Input: part model. Units: mm. Frame: model coordinates. Face numbers are marked on the shaded views. Coordinates: 2 decimals unless noted, no trailing zeros. Order: outer loops, then holes, each group sorted by start corner. A loop starts at its lowest first (then second) coordinate and runs counter-clockwise, first axis right, second up. Notation, with made-up numbers: (69, -31) - (93, -31) arc R21 ccw to (93, -22) - close; hole circle Ø5 at (57.5, 35.5). An arc over 180 degrees is marked (long way). Use a Markdown table: item, result. Add a question column.
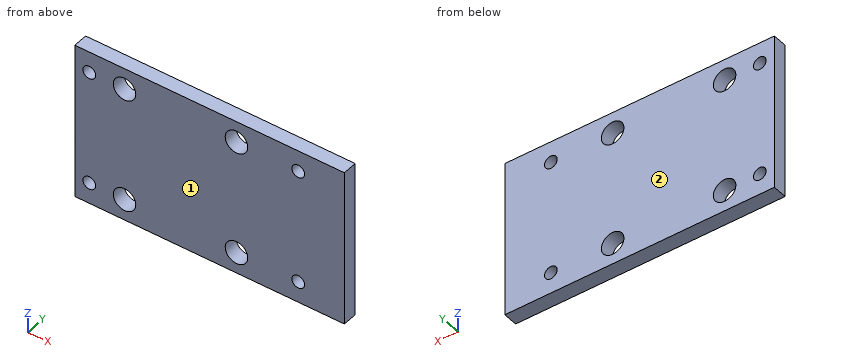
from build123d import *

# Parameters (mm, degrees)
SKETCH1_W           = 74.2
SKETCH1_H           = 46
BOSS_EXTRUDE1_DEPTH = 43
SKETCH2_R           = 11.5
SKETCH2_R_2         = 1.75
SKETCH2_R_3         = 2.5
CUT_EXTRUDE1_DEPTH  = 20
SKETCH3_R           = 3.1
SKETCH3_R_2         = 1.75
CUT_EXTRUDE2_DEPTH  = 15
CUT_EXTRUDE3_DEPTH  = 2.4
SKETCH5_R           = 2.75
CUT_EXTRUDE4_DEPTH  = 12.4


with BuildPart() as part:
    # Sketch1 → Boss-Extrude1 (new body)
    with BuildSketch(Plane.XY):
        with Locations((-13.1, 10)):
            Rectangle(SKETCH1_W, SKETCH1_H)
        Polygon((0, 0), (20, 0), (20, 20), (0, 20), (0, 29), (-42.2, 29), (-42.2, -9), (0, -9), align=None, mode=Mode.SUBTRACT)
    extrude(amount=BOSS_EXTRUDE1_DEPTH)

    # Sketch2 → Cut-Extrude1 (cut)
    with BuildSketch(Plane.XZ.offset(13)):
        with Locations((-21.1, 21.5)):
            Circle(SKETCH2_R)
        with Locations((-36.509600894, 37.201726029)):
            Circle(SKETCH2_R_2)
        with Locations((-5.690399106, 5.798273971)):
            Circle(SKETCH2_R_2)
        with Locations((-36.509600894, 5.798273971)):
            Circle(SKETCH2_R_2)
        with Locations((-5.690399106, 37.201726029)):
            Circle(SKETCH2_R_2)
        with Locations((10, 37.201726029)):
            Circle(SKETCH2_R_3)
        with Locations((10, 5.798273971)):
            Circle(SKETCH2_R_3)
    extrude(amount=-CUT_EXTRUDE1_DEPTH, mode=Mode.SUBTRACT)

    # Sketch3 → Cut-Extrude2 (cut)
    with BuildSketch(Plane(origin=(0, 33, 0), x_dir=(1, 0, 0), z_dir=(0, 1, 0))):
        with Locations(Location((-36.509600894, -5.798273971, 0), (0, 0, 270))):
            Circle(SKETCH3_R)
        with Locations(Location((-5.690399106, -5.798273971, 0), (0, 0, 270))):
            Circle(SKETCH3_R)
        with Locations(Location((-5.690399106, -37.201726029, 0), (0, 0, 270))):
            Circle(SKETCH3_R)
        with Locations(Location((-36.509600894, -37.201726029, 0), (0, 0, 270))):
            Circle(SKETCH3_R)
        with Locations(Location((-46.2, -5.798273971, 0), (0, 0, 270))):
            Circle(SKETCH3_R_2)
        with Locations(Location((-46.2, -37.201726029, 0), (0, 0, 270))):
            Circle(SKETCH3_R_2)
        with Locations(Location((11.309600894, -5.798273971, 0), (0, 0, 270))):
            Circle(SKETCH3_R_2)
        with Locations(Location((11.309600894, -37.201726029, 0), (0, 0, 270))):
            Circle(SKETCH3_R_2)
    extrude(amount=-CUT_EXTRUDE2_DEPTH, mode=Mode.SUBTRACT)


with BuildPart() as body_2:
    # Split1: the piece on the far side of the plane
    add(part.part)
    split(bisect_by=Plane.ZX.offset(29), keep=Keep.BOTTOM)

    # Sketch4 → Cut-Extrude3 (cut)
    with BuildSketch(Plane(origin=(0, 29, 0), x_dir=(1, 0, 0), z_dir=(0, 1, 0))):
        Polygon((-46.2, -2.334172356), (-49.2, -4.066223163), (-49.2, -7.530324778), (-46.2, -9.262375586), (-43.2, -7.530324778), (-43.2, -4.066223163), align=None)
        Polygon((-43.2, -35.469675222), (-46.2, -33.737624414), (-49.2, -35.469675222), (-49.2, -38.933776837), (-46.2, -40.665827644), (-43.2, -38.933776837), align=None)
        Polygon((14.309600894, -4.066223163), (11.309600894, -2.334172356), (8.309600894, -4.066223163), (8.309600894, -7.530324778), (11.309600894, -9.262375586), (14.309600894, -7.530324778), align=None)
        Polygon((14.309600894, -35.469675222), (11.309600894, -33.737624414), (8.309600894, -35.469675222), (8.309600894, -38.933776837), (11.309600894, -40.665827644), (14.309600894, -38.933776837), align=None)
    extrude(amount=-CUT_EXTRUDE3_DEPTH, mode=Mode.SUBTRACT)

    # Sketch5 → Cut-Extrude4 (cut)
    with BuildSketch(Plane(origin=(24, 0, 0), x_dir=(0, 0, -1), z_dir=(1, 0, 0))):
        with Locations(Location((-35.5, 10, 0), (0, 0, 90))):
            Circle(SKETCH5_R)
        with Locations(Location((-7.5, 10, 0), (0, 0, 90))):
            Circle(SKETCH5_R)
    extrude(amount=-CUT_EXTRUDE4_DEPTH, mode=Mode.SUBTRACT)


with BuildPart() as part_1:
    add(part.part)

    # Split1
    split(bisect_by=Plane.ZX.offset(29), keep=Keep.TOP)


solid = part_1.part
1) Contact query for a flat-ended pin moving along its axis: P1, Ø8, axis at x = -5.69, z = 5.8, coming from the -Y side. Output: stop coordinate, or through.
2) Material intervals for L1, parallel to X at y = 31.2, z = 38.5; L2, parallel to X at y = 29.35, z = 3; L3, parallel to X at y = 32.05, z = 4, sorted ascending.
3) Cut plane A-A (x = -46.2). Return the cut outline in (y, z), and give its area (3 significant figures).
4) Cut plane B-B (y = 30.9). State how many separate pieces and enclosed holes the cut face has, and give its area (3 significant figures).
5) Pull-direction query (Y, two-part tool) for the marked faces 1 and 2; classes: pulls with the +Y half, pulls with the -Y half, needs draft (parallel to the pull), parting line crosses it, or undercut.
Computed:
| question | item | result |
|---|---|---|
| 1 | P1 | stops at y = 29 |
| 2 | L1 | x = -50.2 to -47.37, -45.03 to -39.32, -33.69 to -8.51, -2.88 to 10.14, 12.48 to 24 |
| 2 | L2 | x = -50.2 to -37.84, -35.18 to -7.02, -4.36 to 24 |
| 2 | L3 | x = -50.2 to -39.03, -33.98 to -8.22, -3.17 to 24 |
| 3 | outline | (29, 0) - (33, 0) - (33, 4.05) - (29, 4.05) - close; (29, 7.55) - (33, 7.55) - (33, 35.45) - (29, 35.45) - close; (29, 38.95) - (33, 38.95) - (33, 43) - (29, 43) - close |
| 3 | area | 144 mm2 |
| 4 | separate pieces | 1 |
| 4 | enclosed holes | 8 |
| 4 | area | 3,030 mm2 |
| 5 | face 1 | pulls with the -Y half |
| 5 | face 2 | pulls with the +Y half |
